Check sheet for the modelled part. Datum: model origin and axes. Units: mm. Round coordinates to 2 decimals unless told otherwise and drop trailing zeros. Order: outer loops, then holes, each group sorted by start corner. A loop starts at its lowest first (then second) coordinate and runs counter-clockwise, first axis right, second up. Notation, with made-up numbers: (-5, -34) -> (6, -34) arc R18 ccw to (6, -22) -> close; hole circle Ø8 at (-15.75, 61.5). An arc over 180 degrees is marked (long way). Answer in a Markdown table with one row per item.
from build123d import *

# Parameters (mm, degrees)
F0_R     = 16.25
F1_DEPTH = 2.5
F2_R     = 15.05
F3_DEPTH = 2.501
F4_SIZE2 = 0.4618802154
F4_SIZE  = 0.8
F5_SIZE2 = 0.2309401077
F5_SIZE  = 0.4


with BuildPart() as f1:
    # F0 (on Top) → F1 (new body)
    with BuildSketch(Plane.XY):
        Circle(F0_R)
    extrude(amount=F1_DEPTH)

    # F2 (on face) → F3 (cut, through all)
    with BuildSketch(Plane.XY.offset(2.5)):
        Circle(F2_R)
    extrude(amount=-F3_DEPTH, mode=Mode.SUBTRACT)

    # F4
    f4_edges = [f1.edges().sort_by_distance(p)[0] for p in [
        (-15.05, 0, 2.5),
        (-15.05, 0, 0),
    ]]
    f4_side = f1.faces().sort_by_distance((-15.05, 0, 1.25))[0]
    chamfer(f4_edges, length=F4_SIZE, length2=F4_SIZE2, reference=f4_side)

    # F5
    f5_edges = [f1.edges().sort_by_distance(p)[0] for p in [
        (-16.25, 0, 0),
    ]]
    f5_side = f1.faces().sort_by_distance((-16.25, 0, 1.25))[0]
    chamfer(f5_edges, length=F5_SIZE, length2=F5_SIZE2, reference=f5_side)


solid = f1.part
Item 1: Mould release check, pull along X, two halves, no side actions. Record for faces 1 (the cylindrical face through (-3.263, -14.692, 1.256)), 2 (the flat face through (0, -16, 2.5)), 3 (the cylindrical face through (15.5, 4.88, 1.44)): pulls with the +X half, pulls with the -X half, needs draft (parallel to the pull), parting line crosses it, or undercut.
Result sheet:
| item | result |
|---|---|
| face 1 | undercut |
| face 2 | needs draft |
| face 3 | parting line crosses it |
Item 2: Scan lines: line 1 (X direction, y = 0.5, z = 0.9); line 2 (Y direction, x = 0, z = 1); line 3 (X direction, y = 12.5, z = 2.2). Record each from-to range of solid material in increasing order. Write a range as [from, to].
Result sheet:
| item | result |
|---|---|
| line 1 | x = [-16.24, -15.04], [15.04, 16.24] |
| line 2 | y = [-16.25, -15.05], [15.05, 16.25] |
| line 3 | x = [-10.38, -8.89], [8.89, 10.38] |
Item 3: Depth check by flat-ended pin: P1, Ø1.5, axis at x = -4.5, z = 1, coming from the -Y side; P2, Ø18, axis at x = 0, y = 0, coming from the -Z side; P3, Ø1.5, axis at x = 11.5, z = 0.5, coming from the +Y side. Enter the tip coordinate at first touch or a pass-through.
Result sheet:
| item | result |
|---|---|
| P1 | stops at y = -15.81 |
| P2 | passes through |
| P3 | stops at y = 12.19 |
Item 4: Cross-section at A-A (x = 0). Record the boundary of the cut face in (y, z).
Result sheet:
| item | result |
|---|---|
| outline | (-16.25, 0.4) -> (-16.02, 0) -> (-15.51, 0) -> (-15.05, 0.8) -> (-15.05, 1.7) -> (-15.51, 2.5) -> (-16.25, 2.5) -> close; (15.05, 0.8) -> (15.51, 0) -> (16.02, 0) -> (16.25, 0.4) -> (16.25, 2.5) -> (15.51, 2.5) -> (15.05, 1.7) -> close |
